Autodesk Inventor part; units mm, degrees
ref_plane "MSC_PF1" through (0, 0, 0) normal (1, 0, 0) x (0, 1, 0)
ref_plane "MSC_PT1" through (0, 0, 0) normal (1, 0, 0) x (0, 1, 0)
ref_plane "YZ Plane" through (0, 0, 0) normal (1, 0, 0) x (0, 1, 0)
sketch "Skizze1" plane through (0, 0, 0) normal (0, 1, 0) x (-1, 0, 0)
  point P0 (0, 0)
sketch "Skizze2" plane through (0, 0, 0) normal (0, 0, 1) x (-1, 0, 0)
  line L0 (-10, 2) -> (-10, 0)
  line L1 (-2.3, 2) -> (-10, 2)
  line L2 (-0.3, 4) -> (-2.3, 2)
  line L3 (0, 4) -> (-0.3, 4)
  line L4 (0, 0) -> (0, 4)
  line L5 (-10, 0) -> (0, 0)
  line L6 (-10, 0) -> (0, 0)
  line L7 (0, -9.6) -> (0, 1.6)
  line L8 (2, 0) -> (-12, 0)
  dimension "ParC" = 0.3
  dimension "d43" = 45
  dimension "d44" = 4
  dimension "d45" = 2
  dimension "d46" = 10
  dimension "d47" = 0
  dimension "d48" = 0
revolve "Drehung1" add sketch "Skizze2" angle 360 about axis through (10, 0, 0) along (1, 0, 0)
sketch "Skizze3" plane through (0, 0, 0) normal (-1, 0, 0) x (0, 0, 1)
  line L0 (-1.25, 0.7217) -> (-1.25, -0.7217)
  line L1 (0, 1.4434) -> (-1.25, 0.7217)
  line L2 (1.25, 0.7217) -> (0, 1.4434)
  line L3 (1.25, -0.7217) -> (1.25, 0.7217)
  line L4 (0, -1.4434) -> (1.25, -0.7217)
  line L5 (-1.25, -0.7217) -> (0, -1.4434)
  circle A0 centre (0, 0) radius 1.25 construction
  circle A1 centre (0, 0) radius 2 construction
  dimension "d11" = 2.5
  dimension "d13" = 120
  dimension "d15" = 120
extrude "Extrusion1" cut sketch "Skizze3" against normal blind 1.8
fillet "Rundung1" radius 0.2 1 edges at (2.3, 2, 0)
chamfer "Fase1" distance 0.35 angle 45 1 edges at (10, 2, 0) measured on face at (7.4609, 0.9288, -1.7713)
thread "Gewinde1"
ref_plane "MSC_PF1" through (0, 0, 0) normal (1, 0, 0) x (0, 1, 0)
ref_plane "MSC_PT1" through (0, 0, 0) normal (1, 0, 0) x (0, 1, 0)
equation "\"d43\" = 0.5 * ang"
equation "\"d44\" = 0.5 * dk"
equation "\"d45\" = 0.5 * NND"
equation "\"d46\" = NLG"
equation "\"d11\" = ParS"
equation "\"d16\" = ParT"
equation "\"d18\" = r"
equation "\"d19\" = 0.5 * PTC"
equation "\"d39\" = 0.5 * PTC"
equation "\"NND\" = 4"
equation "\"PTC\" = 0.7"
equation "\"dk\" = 8"
equation "\"ParK\" = 2.3"
equation "\"ParS\" = 2.5"
equation "\"ParT\" = 1.8"
equation "\"r\" = 0.2"
equation "\"NLG\" = 10"
equation "\"ang\" = 90deg"
equation "\"THREADDIA\" = NND"
properties part number "ISO 10642 - M4 x  10" material "Stahl"
Source: CAD feature listing. Evaluate the final solid. Frame: model axes, mm. A direction names the side the tool comes from. Coordinates: 2 decimals unless noted, no trailing zeros. Loops run counter-clockwise (first coordinate to the right, second up) from the corner with the lowest first, then second, coordinate; pieces in that order, holes last. Notation, with made-up numbers: M 40,-29.75 L 77,-29.75 A9 ccw 77,-18.75 Z; hole C 52.25,-24 d11. An arc over 180 degrees is marked long. Use a Markdown table: item, result. Add a question column.
Q1. Material intervals for L1, parallel to Y at x = 1.5, z = 1; L2, parallel to X at y = 1, z = -0.25; L3, parallel to Z at x = 0.75, y = -0.5, sorted ascending.
Q2. Access query for faces 4 (the flat face through (1, 0, 1.25)), 5 (the flat face through (0, -2, 0)), 6 (the cylindrical face through (6, 0, 2)). Directions: +Z, -Z, +X, -X, +Y, -Y. A direction counts if a zero-diameter tool reaches every point of the face in a straight line with its end or side. Return the directions, or none.
Q3. First-contact query: pin 1 (4 mm diameter, centred on x = 8, y = 0.5, fed in from +Z); pin 2 (4 mm diameter, centred on x = 2, z = 3, fed in from +Y); pin 3 (0.7 mm diameter, centred on x = 1, y = 0, fed in from +Z). Flat tips, straight axial feed; report the tip coordinate or a pass-through.
Q4. Draft query along Z for faces 1 (the flat face through (10, 0, 0)), 2 (the flat face through (0.89, -1.08, -0.63)), 3 (the conical face through (2.1, 2.2, 0.1)). Return one class per face: pulls with the +Z half, pulls with the -Z half, needs draft (parallel to the pull), parting line crosses it, or undercut.
Q5. Section query A-A, the plane x = 9. Return loops of the section in (y, z), and give its area (3 significant figures).
Result:
| question | item | result |
|---|---|---|
| 1 | L1 | y = -2.62 to -0.87, 0.87 to 2.62 |
| 1 | L2 | x = 1.8 to 10 |
| 1 | L3 | z = -3.51 to -1.25, 1.25 to 3.51 |
| 2 | face 4 | -X |
| 2 | face 5 | +Z, -Z, -X, +Y, -Y |
| 2 | face 6 | +X |
| 3 | pin 1 | stops at z = 2 |
| 3 | pin 2 | stops at y = 3.49 |
| 3 | pin 3 | stops at z = 3.65 |
| 4 | face 1 | needs draft |
| 4 | face 2 | undercut |
| 4 | face 3 | parting line crosses it |
| 5 | outline | C 0,0 d4 |
| 5 | area | 12.6 mm2 |
